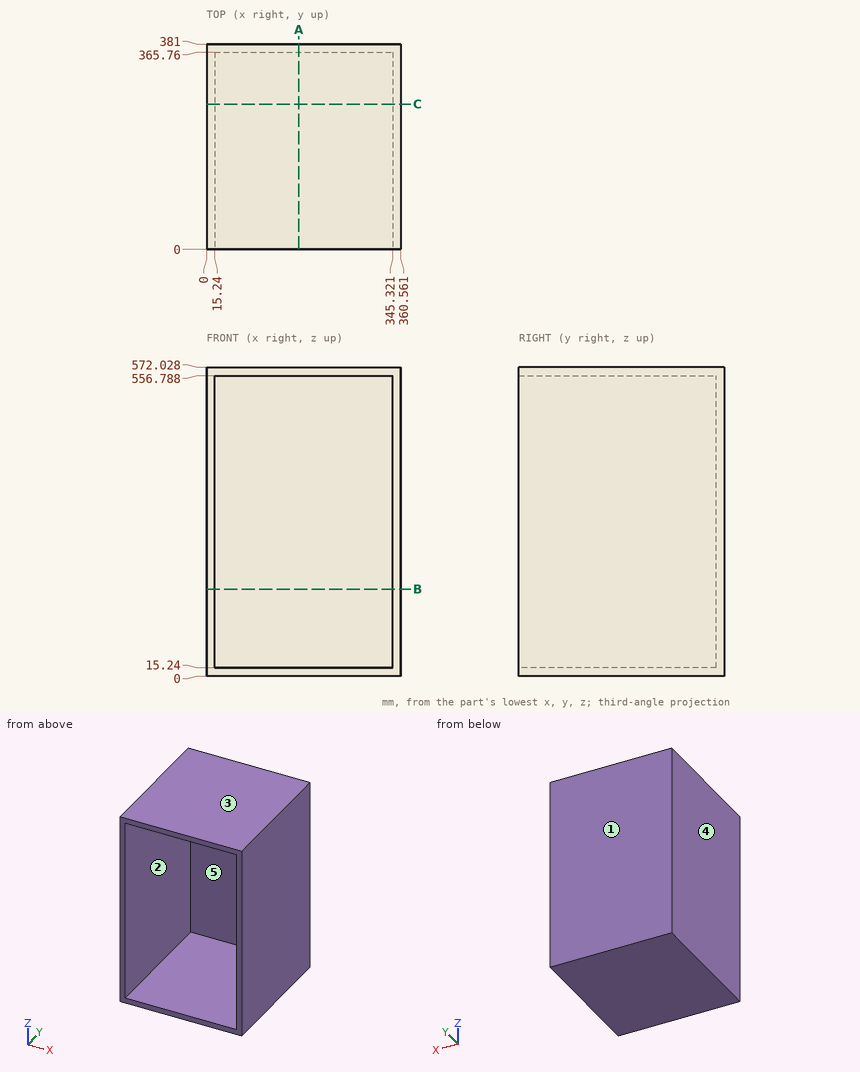
Here's the drawing with two shaded views (mm, measured from the low corner). I have some questions. A direction names the side the tool comes from. Round coordinates to 2 decimals unless told otherwise and drop trailing zeros. Loops run counter-clockwise (first coordinate to the right, second up) from the corner with the lowest first, then second, coordinate; pieces in that order, holes last. Notation, with made-up numbers: (78, 14.25) - (97, 14.25) arc R7 ccw to (97, 24.25) - close; hole circle Ø4 at (44, 32). An arc over 180 degrees is marked (long way). Use CSV: the item, a comma, the result in double quotes. Start each with the question number.
1) For the marked faces 1 and 2, which set-ups out of +Z, -Z, +X, -X, +Y, -Y let a thin tool reach every point of the face, with its end or its side?
2) We'd pull the mould along X, two halves only. Please class the marked faces 3, 4 and 5: released by +X, released by -X, zero draft, split by the parting line, or undercut.
3) If we section it at B-B on z = 161: Write out the boundary of the cut face in (x, y).
4) If we section it at A-A on x = 171: Write out the boundary of the cut face in (y, z).
5) If we section it at C-C on y = 269.5: Write out the boundary of the cut face in (x, z).
6) Please list where these lines run through material, in increasing order: probe 1 along Z at (x, y) = (322.5, 138.5); probe 2 along X at (y, z) = (289.5, 522.5); probe 3 along Y at (x, z) = (131, 517). Write a range as [from, to].
7) For pin 1 Ø4 at (x, z) = (280.5, 265) entering from -Y, with a flat end and sliding along its axis, tell me the tip position at first contact or that it passes through.
Geometry results:
1,face 1,"+Z, -Z, +X, -X, +Y"
1,face 2,"-Y"
2,face 3,"zero draft"
2,face 4,"released by -X"
2,face 5,"undercut"
3,outline,"(0, 0) - (15.24, 0) - (15.24, 365.76) - (345.32, 365.76) - (345.32, 0) - (360.56, 0) - (360.56, 381) - (0, 381) - close"
4,outline,"(0, 0) - (381, 0) - (381, 572.03) - (0, 572.03) - (0, 556.79) - (365.76, 556.79) - (365.76, 15.24) - (0, 15.24) - close"
5,outline,"(0, 0) - (360.56, 0) - (360.56, 572.03) - (0, 572.03) - close; hole (15.24, 15.24) - (345.32, 15.24) - (345.32, 556.79) - (15.24, 556.79) - close"
6,probe 1,"z = [0, 15.24], [556.79, 572.03]"
6,probe 2,"x = [0, 15.24], [345.32, 360.56]"
6,probe 3,"y = [365.76, 381]"
7,pin 1,"stops at y = 365.76"
